Build history of the part. All positions in model axes, mm. A direction names the side the tool comes from. Coordinates: 2 decimals unless noted, no trailing zeros. Order: outer loops, then holes, each group sorted by start corner. A loop starts at its lowest first (then second) coordinate and runs counter-clockwise, first axis right, second up. Notation, with made-up numbers: (-19.5, 26) - (26.5, 26) arc R32 ccw to (26.5, 53) - close; hole circle Ø8 at (1.5, 85). An arc over 180 degrees is marked (long way). Return JSON: item names as keys, results as strings.
from build123d import *

# Parameters (mm, degrees)
SKETCH1_W           = 38.1
SKETCH1_H           = 279.4
BOSS_EXTRUDE1_DEPTH = 19.05
SKETCH2_R           = 6.35
SKETCH2_R_2         = 3.302
CUT_EXTRUDE1_DEPTH  = 20.05
SKETCH3_W           = 34.925
SKETCH3_H           = 12.7
CUT_EXTRUDE2_DEPTH  = 330.2


with BuildPart() as part:
    # Sketch1 → Boss-Extrude1 (new body)
    with BuildSketch(Plane(origin=(0, 0, 0), x_dir=(1, 0, 0), z_dir=(0, 1, 0))):
        with Locations((19.05, 139.7)):
            Rectangle(SKETCH1_W, SKETCH1_H)
        with BuildLine():
            Line((7.9375, 270.66875), (11.1125, 270.66875))
            ThreePointArc((11.1125, 270.66875), (15.08125, 266.7), (11.1125, 262.73125))
            Line((11.1125, 262.73125), (7.9375, 262.73125))
            ThreePointArc((7.9375, 262.73125), (3.96875, 266.7), (7.9375, 270.66875))
        make_face(mode=Mode.SUBTRACT)
        with BuildLine():
            Line((7.9375, 237.33125), (11.1125, 237.33125))
            ThreePointArc((11.1125, 237.33125), (15.08125, 241.3), (11.1125, 245.26875))
            Line((11.1125, 245.26875), (7.9375, 245.26875))
            ThreePointArc((7.9375, 245.26875), (3.96875, 241.3), (7.9375, 237.33125))
        make_face(mode=Mode.SUBTRACT)
        with BuildLine():
            Line((7.9375, 211.93125), (11.1125, 211.93125))
            ThreePointArc((11.1125, 211.93125), (15.08125, 215.9), (11.1125, 219.86875))
            Line((11.1125, 219.86875), (7.9375, 219.86875))
            ThreePointArc((7.9375, 219.86875), (3.96875, 215.9), (7.9375, 211.93125))
        make_face(mode=Mode.SUBTRACT)
        with BuildLine():
            Line((7.9375, 186.53125), (11.1125, 186.53125))
            ThreePointArc((11.1125, 186.53125), (15.08125, 190.5), (11.1125, 194.46875))
            Line((11.1125, 194.46875), (7.9375, 194.46875))
            ThreePointArc((7.9375, 194.46875), (3.96875, 190.5), (7.9375, 186.53125))
        make_face(mode=Mode.SUBTRACT)
        with BuildLine():
            Line((7.9375, 161.13125), (11.1125, 161.13125))
            ThreePointArc((11.1125, 161.13125), (15.08125, 165.1), (11.1125, 169.06875))
            Line((11.1125, 169.06875), (7.9375, 169.06875))
            ThreePointArc((7.9375, 169.06875), (3.96875, 165.1), (7.9375, 161.13125))
        make_face(mode=Mode.SUBTRACT)
        with BuildLine():
            Line((7.9375, 135.73125), (11.1125, 135.73125))
            ThreePointArc((11.1125, 135.73125), (15.08125, 139.7), (11.1125, 143.66875))
            Line((11.1125, 143.66875), (7.9375, 143.66875))
            ThreePointArc((7.9375, 143.66875), (3.96875, 139.7), (7.9375, 135.73125))
        make_face(mode=Mode.SUBTRACT)
        with BuildLine():
            Line((7.9375, 110.33125), (11.1125, 110.33125))
            ThreePointArc((11.1125, 110.33125), (15.08125, 114.3), (11.1125, 118.26875))
            Line((11.1125, 118.26875), (7.9375, 118.26875))
            ThreePointArc((7.9375, 118.26875), (3.96875, 114.3), (7.9375, 110.33125))
        make_face(mode=Mode.SUBTRACT)
        with BuildLine():
            Line((7.9375, 84.93125), (11.1125, 84.93125))
            ThreePointArc((11.1125, 84.93125), (15.08125, 88.9), (11.1125, 92.86875))
            Line((11.1125, 92.86875), (7.9375, 92.86875))
            ThreePointArc((7.9375, 92.86875), (3.96875, 88.9), (7.9375, 84.93125))
        make_face(mode=Mode.SUBTRACT)
        with BuildLine():
            Line((7.9375, 59.53125), (11.1125, 59.53125))
            ThreePointArc((11.1125, 59.53125), (15.08125, 63.5), (11.1125, 67.46875))
            Line((11.1125, 67.46875), (7.9375, 67.46875))
            ThreePointArc((7.9375, 67.46875), (3.96875, 63.5), (7.9375, 59.53125))
        make_face(mode=Mode.SUBTRACT)
        with BuildLine():
            Line((7.9375, 34.13125), (11.1125, 34.13125))
            ThreePointArc((11.1125, 34.13125), (15.08125, 38.1), (11.1125, 42.06875))
            Line((11.1125, 42.06875), (7.9375, 42.06875))
            ThreePointArc((7.9375, 42.06875), (3.96875, 38.1), (7.9375, 34.13125))
        make_face(mode=Mode.SUBTRACT)
        with BuildLine():
            Line((7.9375, 8.73125), (11.1125, 8.73125))
            ThreePointArc((11.1125, 8.73125), (15.08125, 12.7), (11.1125, 16.66875))
            Line((11.1125, 16.66875), (7.9375, 16.66875))
            ThreePointArc((7.9375, 16.66875), (3.96875, 12.7), (7.9375, 8.73125))
        make_face(mode=Mode.SUBTRACT)
    extrude(amount=BOSS_EXTRUDE1_DEPTH)

    # Sketch2 → Cut-Extrude1 (cut, through all)
    with BuildSketch(Plane(origin=(0, 19.05, 0), x_dir=(1, 0, 0), z_dir=(0, 1, 0))):
        with Locations((25.4, 230.414285714)):
            Circle(SKETCH2_R)
        with Locations((25.4, 194.128571429)):
            Circle(SKETCH2_R)
        with Locations((25.4, 157.842857143)):
            Circle(SKETCH2_R)
        with Locations((25.4, 121.557142857)):
            Circle(SKETCH2_R)
        with Locations((25.4, 85.271428571)):
            Circle(SKETCH2_R)
        with Locations((25.4, 48.985714286)):
            Circle(SKETCH2_R)
        with Locations((25.4, 266.7)):
            Circle(SKETCH2_R_2)
        with Locations((25.4, 12.7)):
            Circle(SKETCH2_R_2)
    extrude(amount=-CUT_EXTRUDE1_DEPTH, mode=Mode.SUBTRACT)

    # Sketch3 → Cut-Extrude2 (cut)
    with BuildSketch(Plane.XY):
        with Locations((20.6375, 9.525)):
            Rectangle(SKETCH3_W, SKETCH3_H)
    extrude(amount=-CUT_EXTRUDE2_DEPTH, mode=Mode.SUBTRACT)


solid = part.part
1. Cut at A-A on z = -12.7. Give the cut face in (x, y) (3 decimals).
Check values:
{"outline": "(0, 0) - (3.969, 0) - (3.969, 3.175) - (3.175, 3.175) - (3.175, 15.875) - (3.969, 15.875) - (3.969, 19.05) - (0, 19.05) - close; (15.081, 0) - (22.098, 0) - (22.098, 3.175) - (15.081, 3.175) - close; (15.081, 15.875) - (22.098, 15.875) - (22.098, 19.05) - (15.081, 19.05) - close; (28.702, 0) - (38.1, 0) - (38.1, 3.175) - (28.702, 3.175) - close; (28.702, 15.875) - (38.1, 15.875) - (38.1, 19.05) - (28.702, 19.05) - close"}
2. Cut at D-D on y = 11.25. Give the cut face in (x, z) (3 decimals).
Check values:
{"outline": "(0, -279.4) - (3.175, -279.4) - (3.175, 0) - (0, 0) - close"}
3. Mould opens along X. For faces 3 (the flat face through (15, 3, 0)), 4 (the flat face through (3.175, 9, -138)), 5 (the cylindrical face through (19.056, 17.485, -49.265)), 6 (the cylindrical face through (24.57, 1.61, -236.71)) say: pulls with the +X half, pulls with the -X half, needs draft (parallel to the pull), parting line crosses it, or undercut.
Check values:
{"face 3": "needs draft", "face 4": "pulls with the +X half", "face 5": "undercut", "face 6": "undercut"}
4. Cut at B-B on z = -215.9. Give the cut face in (x, y) (3 decimals), plus the area to 3 significant figures.
Check values:
{"outline": "(0, 0) - (3.969, 0) - (3.969, 3.175) - (3.175, 3.175) - (3.175, 15.875) - (3.969, 15.875) - (3.969, 19.05) - (0, 19.05) - close; (15.081, 0) - (38.1, 0) - (38.1, 3.175) - (15.081, 3.175) - close; (15.081, 15.875) - (38.1, 15.875) - (38.1, 19.05) - (15.081, 19.05) - close", "area": "212 mm²"}
5. Tool access for faces 1 (the cylindrical face through (24.97, 17.485, -269.974)), 2 (the flat face through (20, 3.175, -138)): list every direction of +Z, -Z, +X, -X, +Y, -Y with a clear straight run to the whole face (end or side of a thin tool).
Check values:
{"face 1": "+Y, -Y", "face 2": "+Z, -Z, +X"}
6. Drop a flat-ended pin along its axis: pin 1 (10 mm diameter, centred on x = 25.4, z = -48.99, fed in from -Y). Give the stop position or say it passes through.
Check values:
{"pin 1": "through"}
7. Cut at C-C on x = 25.4. State how many separate pieces and enclosed holes the cut face has, plus the area to 3 significant figures.
Check values:
{"separate pieces": "18", "enclosed holes": "0", "area": "1,210 mm²"}
8. Probe L1, parallel to X at y = 2.4, z = -266.7; L2, parallel to Y at x = 33, z = -161 (3 decimals); L3, parallel to X at y = 11.25, z = -28 (3 decimals). List the from-to ranges inside material, lowest first.
Check values:
{"L1": "0 to 3.97, 15.08 to 22.1, 28.7 to 38.1", "L2": "0 to 3.175, 15.875 to 19.05", "L3": "0 to 3.175"}
